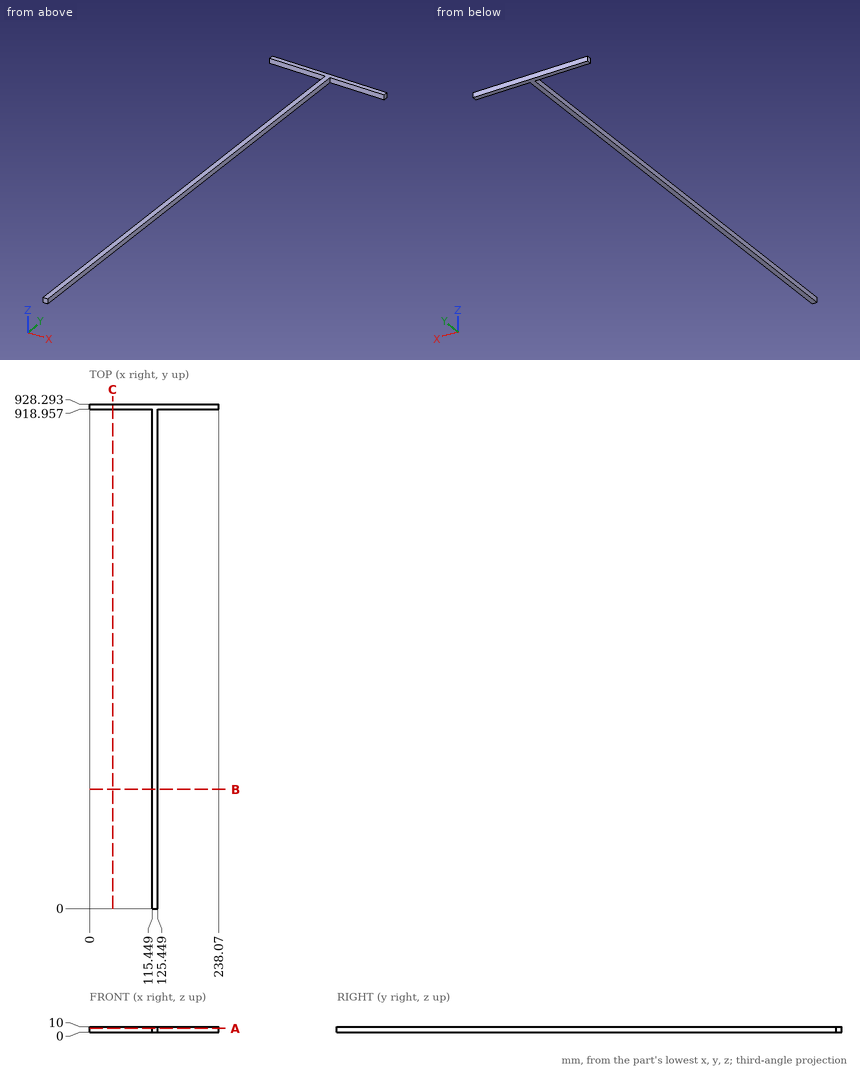
Part print with two shaded views. Sizes in mm from the minimum x, y, z corner. Round coordinates to 2 decimals unless told otherwise and drop trailing zeros. Write each loop counter-clockwise with the first axis right and the second up, starting at its lowest first coordinate (ties: lowest second). Pieces come first, ordered by that corner, then holes. Notation, with made-up numbers: (-4.75, 89.5) - (18.25, 89.5) arc R34 ccw to (18.25, 128.5) - close; hole circle Ø11 at (-7, 9.25). An arc over 180 degrees is marked (long way). Answer as CSV lines item,"result".
Q1. Drop flat-ended pins along their axis: pin 1 (1.5 mm diameter, centred on y = 253.5, z = 2, fed in from -X); pin 2 (3 mm diameter, centred on x = 203, z = 4, fed in from -Y). Give the stop position or say it passes through.
Report:
pin 1,"stops at x = 115.45"
pin 2,"stops at y = 918.96"
Q2. Cut at C-C (x = 42.5). Write the cut outline in (y, z).
Report:
outline,"(918.96, 0) - (928.29, 0) - (928.29, 10) - (918.96, 10) - close"
Q3. Cut at B-B (y = 219.5). Write the cut outline in (x, z).
Report:
outline,"(115.45, 0) - (125.45, 0) - (125.45, 10) - (115.45, 10) - close"
Q4. Drill centre lines: probe 1 along Y at (x, z) = (106, 6.5); probe 2 along X at (y, z) = (726, 1). Where is each one in solid material? Low to high. Write a range as [from, to].
Report:
probe 1,"y = [918.96, 928.29]"
probe 2,"x = [115.45, 125.45]"
Q5. Cut at A-A (z = 6.75). Write the cut outline in (x, y).
Report:
outline,"(0, 918.96) - (115.45, 918.96) - (115.45, 0) - (125.45, 0) - (125.45, 918.96) - (238.07, 918.96) - (238.07, 928.29) - (0, 928.29) - close"
